```python
from build123d import *

# Parameters (mm, degrees)
SKETCH1_W           = 67
SKETCH1_H           = 43
BOSS_EXTRUDE1_DEPTH = 8
SKETCH2_W           = 6
SKETCH2_H           = 43
BOSS_EXTRUDE2_DEPTH = 82
CUT_EXTRUDE1_REACH  = 112.83
SKETCH3_R           = 11.25
SKETCH3_R_2         = 1.5
CUT_EXTRUDE2_REACH  = 112.83
SKETCH4_R           = 4.1
FILLET1_R           = 20
SKETCH6_R           = 2.9
CUT_EXTRUDE4_DEPTH  = 4
SKETCH7_R           = 6
CUT_EXTRUDE5_DEPTH  = 3.5
CUT_EXTRUDE6_START  = -8
SKETCH8_R           = 16
CUT_EXTRUDE6_DEPTH  = 3.5
SKETCH9_R           = 2.9
CUT_EXTRUDE7_DEPTH  = 4


with BuildPart() as part:
    # Sketch1 → Boss-Extrude1 (new body)
    with BuildSketch(Plane(origin=(0, 0, 0), x_dir=(1, 0, 0), z_dir=(0, 1, 0))):
        Rectangle(SKETCH1_W, SKETCH1_H)
    extrude(amount=BOSS_EXTRUDE1_DEPTH)

    # Sketch2 → Boss-Extrude2 (add)
    with BuildSketch(Plane(origin=(0, 8, 0), x_dir=(1, 0, 0), z_dir=(0, 1, 0))):
        with Locations((-30.5, 0)):
            Rectangle(SKETCH2_W, SKETCH2_H)
    extrude(amount=BOSS_EXTRUDE2_DEPTH)

    # Sketch3 → Cut-Extrude1 (cut, up to next)
    with BuildSketch(Plane(origin=(-27.5, 0, 0), x_dir=(0, 0, -1), z_dir=(1, 0, 0)), mode=Mode.PRIVATE) as cut_extrude1_sk1:
        with Locations((0, 29)):
            Circle(SKETCH3_R)
    cut_extrude1_tool1 = extrude(cut_extrude1_sk1.sketch, amount=-CUT_EXTRUDE1_REACH, mode=Mode.PRIVATE) & part.part
    # Sketch3 → Cut-Extrude1 (cut, up to next)
    with BuildSketch(Plane(origin=(-27.5, 0, 0), x_dir=(0, 0, -1), z_dir=(1, 0, 0)), mode=Mode.PRIVATE) as cut_extrude1_sk2:
        with Locations((-15.5, 44.5)):
            Circle(SKETCH3_R_2)
    cut_extrude1_tool2 = extrude(cut_extrude1_sk2.sketch, amount=-CUT_EXTRUDE1_REACH, mode=Mode.PRIVATE) & part.part
    # Sketch3 → Cut-Extrude1 (cut, up to next)
    with BuildSketch(Plane(origin=(-27.5, 0, 0), x_dir=(0, 0, -1), z_dir=(1, 0, 0)), mode=Mode.PRIVATE) as cut_extrude1_sk3:
        with Locations((15.5, 44.5)):
            Circle(SKETCH3_R_2)
    cut_extrude1_tool3 = extrude(cut_extrude1_sk3.sketch, amount=-CUT_EXTRUDE1_REACH, mode=Mode.PRIVATE) & part.part
    # Sketch3 → Cut-Extrude1 (cut, up to next)
    with BuildSketch(Plane(origin=(-27.5, 0, 0), x_dir=(0, 0, -1), z_dir=(1, 0, 0)), mode=Mode.PRIVATE) as cut_extrude1_sk4:
        with Locations((15.5, 13.5)):
            Circle(SKETCH3_R_2)
    cut_extrude1_tool4 = extrude(cut_extrude1_sk4.sketch, amount=-CUT_EXTRUDE1_REACH, mode=Mode.PRIVATE) & part.part
    # Sketch3 → Cut-Extrude1 (cut, up to next)
    with BuildSketch(Plane(origin=(-27.5, 0, 0), x_dir=(0, 0, -1), z_dir=(1, 0, 0)), mode=Mode.PRIVATE) as cut_extrude1_sk5:
        with Locations((-15.5, 13.5)):
            Circle(SKETCH3_R_2)
    cut_extrude1_tool5 = extrude(cut_extrude1_sk5.sketch, amount=-CUT_EXTRUDE1_REACH, mode=Mode.PRIVATE) & part.part
    add(cut_extrude1_tool1.solids().sort_by_distance((-27.5, 29, 0))[0], mode=Mode.SUBTRACT)
    add(cut_extrude1_tool2.solids().sort_by_distance((-27.5, 44.5, 15.5))[0], mode=Mode.SUBTRACT)
    add(cut_extrude1_tool3.solids().sort_by_distance((-27.5, 44.5, -15.5))[0], mode=Mode.SUBTRACT)
    add(cut_extrude1_tool4.solids().sort_by_distance((-27.5, 13.5, -15.5))[0], mode=Mode.SUBTRACT)
    add(cut_extrude1_tool5.solids().sort_by_distance((-27.5, 13.5, 15.5))[0], mode=Mode.SUBTRACT)

    # Sketch4 → Cut-Extrude2 (cut, up to next)
    with BuildSketch(Plane(origin=(-27.5, 0, 0), x_dir=(0, 0, -1), z_dir=(1, 0, 0)), mode=Mode.PRIVATE) as cut_extrude2_sk1:
        with Locations((0, 78)):
            Circle(SKETCH4_R)
    cut_extrude2_tool1 = extrude(cut_extrude2_sk1.sketch, amount=-CUT_EXTRUDE2_REACH, mode=Mode.PRIVATE) & part.part
    add(cut_extrude2_tool1.solids().sort_by_distance((-27.5, 78, 0))[0], mode=Mode.SUBTRACT)

    # Fillet1
    fillet1_edges = [part.edges().sort_by_distance(p)[0] for p in [
        (-30.5, 90, -21.5),
        (-30.5, 90, 21.5),
    ]]
    fillet(fillet1_edges, radius=FILLET1_R)

    # Sketch6 → Cut-Extrude4 (cut)
    with BuildSketch(Plane(origin=(33.5, 0, 0), x_dir=(0, 0, -1), z_dir=(1, 0, 0))):
        with Locations((0, 4)):
            Circle(SKETCH6_R)
        with Locations((10, 4)):
            Circle(SKETCH6_R)
        with Locations((-10, 4)):
            Circle(SKETCH6_R)
    extrude(amount=-CUT_EXTRUDE4_DEPTH, mode=Mode.SUBTRACT)

    # Sketch7 → Cut-Extrude5 (cut)
    with BuildSketch(Plane.ZY.offset(33.5)):
        with Locations((0, 78)):
            Circle(SKETCH7_R)
    extrude(amount=-CUT_EXTRUDE5_DEPTH, mode=Mode.SUBTRACT)

    # Sketch8 → Cut-Extrude6 (cut)
    with BuildSketch(Plane(origin=(0, 8, 0), x_dir=(1, 0, 0), z_dir=(0, 1, 0)).offset(CUT_EXTRUDE6_START)):
        with Locations(Location((3, 0, 0), (0, 0, 270))):
            Circle(SKETCH8_R)
    extrude(amount=CUT_EXTRUDE6_DEPTH, mode=Mode.SUBTRACT)

    # Sketch9 → Cut-Extrude7 (cut)
    with BuildSketch(Plane.XZ.offset(-3.5)):
        with Locations(Location((3, 12, 0), (0, 0, 270))):
            Circle(SKETCH9_R)
        with Locations(Location((15, 0, 0), (0, 0, 270))):
            Circle(SKETCH9_R)
        with Locations(Location((3, -12, 0), (0, 0, 270))):
            Circle(SKETCH9_R)
        with Locations(Location((-9, 0, 0), (0, 0, 270))):
            Circle(SKETCH9_R)
    extrude(amount=-CUT_EXTRUDE7_DEPTH, mode=Mode.SUBTRACT)


solid = part.part
```
CAD build for the part. Positions are in the model's coordinates, mm. A direction names the side the tool comes from. Give positions to 0.01 mm unless a question says otherwise; leave off trailing zeros. Order: outer loops, then holes, each group sorted by start corner. A loop starts at its lowest first (then second) coordinate and runs counter-clockwise, first axis right, second up.
(1) Tool access for faces 4 (the cylindrical face through (-31.77, 83.95, -0.78)), 5 (the cylindrical face through (-30.458, 43.036, -15.175)), 6 (the cylindrical face through (31.528, 6.445, -1.559)), 7 (the flat face through (15, 7.5, 0)), 8 (the flat face through (-15, 6, 21.5)): list every direction of +Z, -Z, +X, -X, +Y, -Y with a clear straight run to the whole face (end or side of a thin tool).
(2) Drill centre lines: L1, parallel to Y at x = -28, z = 0; L2, parallel to X at y = 4.8, z = 0; L3, parallel to Y at x = 31.2, z = 0. Where is each one in solid material? Low to high.
(3) Mould opens along Z. For faces 1 (the cylindrical face through (-30.458, 84.297, -15.486)), 2 (the cylindrical face through (-12.62, 1.73, -3.47)), 3 (the flat face through (3, 8, 0)) say: released by +Z, released by -Z, zero draft, split by the parting line, or undercut.
(4) Saw through at C-C, the plane y = 37. Give the cut face in (x, z), then the cut area to 3 significant figures.
(5) Saw through at D-D, the plane x = 7. Give the cut face in (y, z).
(6) Saw through at A-A, the plane z = 0. State how many separate pieces and enclosed holes the cut face has, then the cut area to 3 significant figures.
(7) Flat gauge pins, fed straight in: pin 1 (6.5 mm diameter, centred on x = 3, z = 12, fed in from +Y); pin 2 (2.5 mm diameter, centred on y = 13.5, z = 15.5, fed in from -X); pin 3 (9.5 mm diameter, centred on y = 78, z = 0, fed in from -X); pin 4 (21.5 mm diameter, centred on y = 40.5, z = -9.5, fed in from +X). Where does each tip first touch, or does it go through?
(8) Saw through at B-B, the plane y = 13.5. Give the cut face in (x, z), then the cut area to 3 significant figures.
Results found:
1. face 4: -X
1. face 5: +X, -X
1. face 6: +X
1. face 7: -Y
1. face 8: +Z, +X, -X, +Y, -Y
2. L1: y = 0 to 17.75, 40.25 to 73.9, 82.1 to 90
2. L2: x = -33.5 to -11.9, -6.1 to 12.1, 17.9 to 29.5
2. L3: y = 0 to 1.1, 6.9 to 8
3. face 1: released by -Z
3. face 2: undercut
3. face 3: zero draft
4. outline: (-33.5, -21.5) - (-27.5, -21.5) - (-27.5, -7.91) - (-33.5, -7.91) - close; (-33.5, 7.91) - (-27.5, 7.91) - (-27.5, 21.5) - (-33.5, 21.5) - close
4. area: 163 mm2
5. outline: (0, -21.5) - (8, -21.5) - (8, 21.5) - (0, 21.5) - (0, 15.49) - (3.5, 15.49) - (3.5, -15.49) - (0, -15.49) - close
6. separate pieces: 3
6. enclosed holes: 0
6. area: 649 mm2
7. pin 1: stops at y = 8
7. pin 2: passes through
7. pin 3: stops at x = -30
7. pin 4: stops at x = -27.5
8. outline: (-33.5, -21.5) - (-27.5, -21.5) - (-27.5, -17) - (-33.5, -17) - close; (-33.5, -14) - (-27.5, -14) - (-27.5, 14) - (-33.5, 14) - close; (-33.5, 17) - (-27.5, 17) - (-27.5, 21.5) - (-33.5, 21.5) - close
8. area: 222 mm2
